```python
from build123d import *

# Parameters (mm, degrees)
F2_R     = 117.132318
F3_DEPTH = 157.902554


with BuildPart() as f1:
    # F0 (on Front) → F1 (revolve)
    with BuildSketch(Plane.XZ):
        with BuildLine():
            Line((0, 20), (20, 20))
            Line((20, 20), (65.331466, 20))
            Line((65.331466, 20), (65.331466, 44.863343))
            Line((65.331466, 44.863343), (20, 44.863343))
            Line((20, 44.863343), (5.857864, 39.005479))
            ThreePointArc((5.857864, 39.005479), (1.522409, 32.517012), (0, 24.863343))
            Line((0, 24.863343), (0, 20))
        make_face()
        with BuildLine():
            Line((65.331466, 44.863343), (65.331466, 20))
            Line((65.331466, 20), (69.630553, 27.648209))
            ThreePointArc((69.630553, 27.648209), (66.667779, 38.217287), (77.236857, 41.180061))
            Line((77.236857, 41.180061), (81.535943, 48.82827))
            Line((81.535943, 48.82827), (69.382586, 48.82827))
            Line((69.382586, 48.82827), (65.331466, 44.863343))
        make_face()
    revolve(axis=Axis((10, 0, 0), (-1, 0, 0)))

    # F2 (on Right) → F3 (cut)
    with BuildSketch(Plane.YZ):
        Circle(F2_R)
        Polygon((-51.961524, 0), (-25.980762, 45), (25.980762, 45), (51.961524, 0), (25.980762, -45), (-25.980762, -45), align=None, mode=Mode.SUBTRACT)
    extrude(amount=F3_DEPTH, mode=Mode.SUBTRACT)


solid = f1.part
```
Source: CAD feature listing. Evaluate the final solid. Frame: model axes, mm. A direction names the side the tool comes from. Round coordinates to 2 decimals unless told otherwise and drop trailing zeros. Order: outer loops, then holes, each group sorted by start corner. A loop starts at its lowest first (then second) coordinate and runs counter-clockwise, first axis right, second up. Notation, with made-up numbers: (71.25, 10) -> (110.25, 10) arc R24 cw to (110.25, 47) -> close; hole circle Ø7 at (6, 88.25). An arc over 180 degrees is marked (long way). One line per item, written item: value. Start each with the question number.
Q1. Section query B-B (y = 0). Return the cut outline in (x, z), plus the area to 3 significant figures.
Q2. Access query for faces 4 (the cylindrical face through (75.374, 24.488, -42.244)), 5 (the cylindrical face through (42.3, -27.3, -35.6)). Directions: +Z, -Z, +X, -X, +Y, -Y. A direction counts if a zero-diameter tool reaches every point of the face in a straight line with its end or side. Return the directions, or none.
Q3. Section query C-C (x = 22.5). Return the cut outline in (y, z), plus the area to 3 significant figures.
Q4. Draft query along Y for faces 1 (the cylindrical face through (33.123, -19.524, -4.336)), 2 (the conical face through (65.64, -44.09, -9.79)), 3 (the flat face through (73.391, 39.104, -22.27)). Return one class per face: pulls with the +Y half, pulls with the -Y half, needs draft (parallel to the pull), parting line crosses it, or undercut.
Q5. Material intervals for probe 1 along Z at (x, y) = (69, 18); probe 2 along Y at (x, z) = (30, 0); probe 3 along Y at (x, z) = (67, -4.5), sorted ascending.
Q6. Pin query (flat end, axial travel): pin 1 (5 mm diameter, centred on x = 18, y = 38.5, fed in from -Z); pin 2 (2 mm diameter, centred on x = 41, z = 11, fed in from -Y); pin 3 (2 mm diameter, centred on x = 12.5, z = 22.5, fed in from +Y). Return the tip coordinate at first contact, or that it passes through.
Q7. Section query A-A (z = 0). Return the cut outline in (x, y).
Findings below:
1. outline: (0, -24.86) arc R20 ccw to (5.86, -39.01) -> (20, -44.86) -> (65.33, -44.86) -> (65.47, -45) -> (79.38, -45) -> (77.24, -41.18) arc R7.76 cw to (69.63, -27.65) -> (65.33, -20) -> (0, -20) -> close; (0, 20) -> (65.33, 20) -> (69.63, 27.65) arc R7.76 cw to (77.24, 41.18) -> (79.38, 45) -> (65.47, 45) -> (65.33, 44.86) -> (20, 44.86) -> (5.86, 39.01) arc R20 ccw to (0, 24.86) -> close
1. area: 3,210 mm²
2. face 4: -Z, +X, -X, +Y
2. face 5: -X
3. outline: circle Ø89.73 at (0, 0); hole circle Ø40 at (0, 0)
3. area: 5,070 mm²
4. face 1: undercut
4. face 2: parting line crosses it
4. face 3: pulls with the +Y half
5. probe 1: -44.99 to -36.6, -21.5 to -19.48, 19.48 to 21.5, 36.6 to 44.99
5. probe 2: -44.86 to -20, 20 to 44.86
5. probe 3: -46.28 to -38.49, -29.73 to -22.52, 22.52 to 29.73, 38.49 to 46.28
6. pin 1: z = -25.79
6. pin 2: y = -43.73
6. pin 3: y = 35.97
7. outline: (0, -24.86) arc R20 ccw to (5.86, -39.01) -> (20, -44.86) -> (65.33, -44.86) -> (69.38, -48.83) -> (81.54, -48.83) -> (77.24, -41.18) arc R7.76 cw to (69.63, -27.65) -> (65.33, -20) -> (0, -20) -> close; (0, 20) -> (65.33, 20) -> (69.63, 27.65) arc R7.76 cw to (77.24, 41.18) -> (81.54, 48.83) -> (69.38, 48.83) -> (65.33, 44.86) -> (20, 44.86) -> (5.86, 39.01) arc R20 ccw to (0, 24.86) -> close
